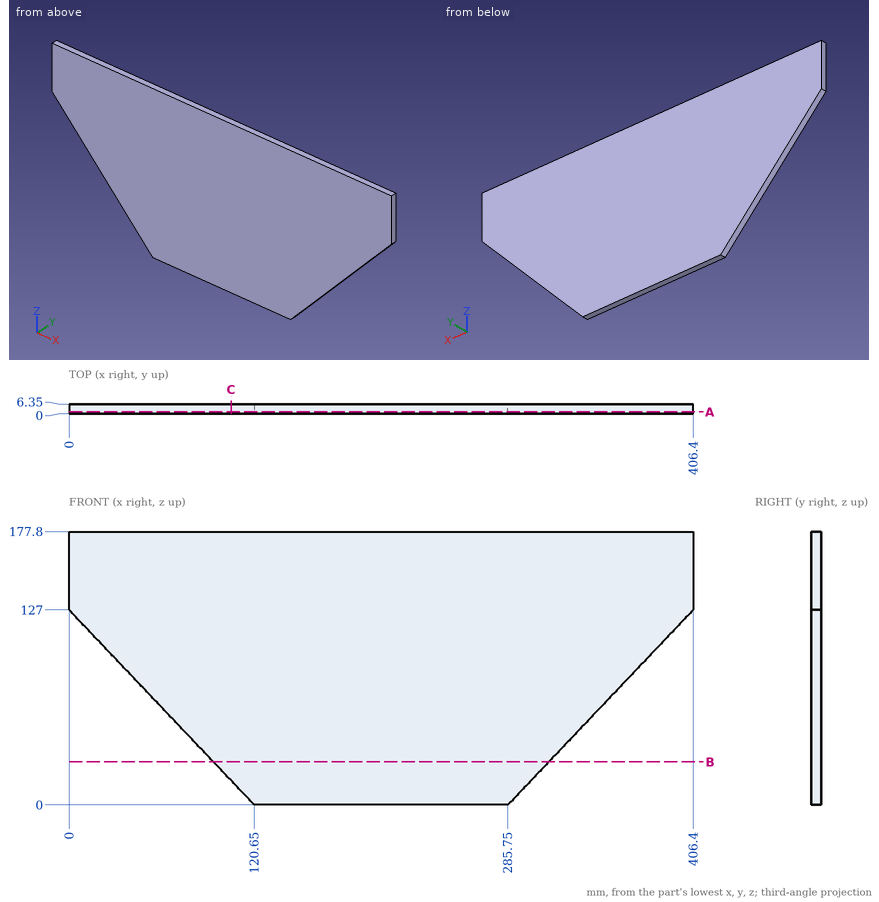
Study the drawing (mm; zero at the part's minimum x, y, z) and answer. Coordinates: 2 decimals unless noted, no trailing zeros. Write each loop counter-clockwise with the first axis right and the second up, starting at its lowest first coordinate (ties: lowest second). Pieces come first, ordered by that corner, then holes. Notation, with made-up numbers: (62.5, -1) - (77.5, -1) arc R18 ccw to (77.5, 23) - close; hole circle Ø1 at (54, 21.25). An arc over 180 degrees is marked (long way). Answer as a JSON object with one key per item and string values. Group by question number.
1. A cutting plane is placed at B-B (z = 28). Determine the outline of the cut face in (x, y).
2. Consider L1, parallel to X at y = 6, z = 60; L2, parallel to X at y = 0.5, z = 35.5 (3 decimals); L3, parallel to Z at x = 47.5, y = 4.25. Determine where each line is inside the solid, lowest interval first. Write a range as [from, to].
3. Each of these flat-tipped pins is pushed along its axis until it touches: P1, Ø1, axis at y = 1, z = 94, coming from the -X side (3 decimals); P2, Ø3, axis at x = 74, y = 0.5, coming from the -Z side. Where does it stop, or does it pass through?
4. A cutting plane is placed at A-A (y = 1.25). Determine the outline of the cut face in (x, z).
5. A cutting plane is placed at C-C (x = 105.5). Determine the outline of the cut face in (y, z), plus the area to 3 significant figures.
Worked out:
{
 "1": {"outline": "(94.05, 0) - (312.35, 0) - (312.35, 6.35) - (94.05, 6.35) - close"},
 "2": {"L1": "x = [63.65, 342.75]", "L2": "x = [86.925, 319.475]", "L3": "z = [77, 177.8]"},
 "3": {"P1": "stops at x = 30.875", "P2": "stops at z = 47.53"},
 "4": {"outline": "(0, 127) - (120.65, 0) - (285.75, 0) - (406.4, 127) - (406.4, 177.8) - (0, 177.8) - close"},
 "5": {"outline": "(0, 15.95) - (6.35, 15.95) - (6.35, 177.8) - (0, 177.8) - close", "area": "1,030 mm²"}
}
